from build123d import *

# Parameters (mm, degrees)
SKETCH_1_W               = 15
SKETCH_1_H               = 15
SKETCH_1_W_2             = 13
SKETCH_1_H_2             = 13
EXTRUDE_1_DEPTH          = 570
CUT_EXTRUDE_1_DEPTH      = 10
CUT_EXTRUDE_1_DEPTH_BACK = 571.098675669
SKETCH_2_R               = 1.45
SKETCH_3_R               = 1.5
CUT_EXTRUDE_2_DEPTH      = 571.246657158


with BuildPart() as part:
    # 草图1 → 拉伸-薄壁1 (new body)
    with BuildSketch(Plane(origin=(0, 0, 0), x_dir=(1, 0, 0), z_dir=(0, 1, 0))):
        Rectangle(SKETCH_1_W, SKETCH_1_H)
        Rectangle(SKETCH_1_W_2, SKETCH_1_H_2, mode=Mode.SUBTRACT)
    extrude(amount=EXTRUDE_1_DEPTH)

    # 草图2 → 切除-拉伸1 (cut, two sides: drawn at the far end of the back side and taken through both)
    with BuildSketch(Plane.XY.offset(-CUT_EXTRUDE_1_DEPTH_BACK)):
        with Locations(Location((0, 7.5, 0), (0, 0, 180))):
            Circle(SKETCH_2_R)
        with Locations(Location((0, 22.5, 0), (0, 0, 180))):
            Circle(SKETCH_2_R)
        with Locations(Location((0, 42.5, 0), (0, 0, 180))):
            Circle(SKETCH_2_R)
        with Locations(Location((0, 527.5, 0), (0, 0, 180))):
            Circle(SKETCH_2_R)
        with Locations(Location((0, 547.5, 0), (0, 0, 180))):
            Circle(SKETCH_2_R)
        with Locations(Location((0, 562.5, 0), (0, 0, 180))):
            Circle(SKETCH_2_R)
        with Locations(Location((0, 285, 0), (0, 0, 180))):
            Circle(SKETCH_2_R)
        with Locations(Location((0, 305, 0), (0, 0, 180))):
            Circle(SKETCH_2_R)
        with Locations(Location((0, 265, 0), (0, 0, 180))):
            Circle(SKETCH_2_R)
        with Locations(Location((0, 190, 0), (0, 0, 180))):
            Circle(SKETCH_2_R)
        with Locations(Location((0, 170, 0), (0, 0, 180))):
            Circle(SKETCH_2_R)
        with Locations(Location((0, 230, 0), (0, 0, 180))):
            Circle(SKETCH_2_R)
        with Locations(Location((0, 210, 0), (0, 0, 180))):
            Circle(SKETCH_2_R)
        with Locations(Location((0, 405, 0), (0, 0, 180))):
            Circle(SKETCH_2_R)
        with Locations(Location((0, 385, 0), (0, 0, 180))):
            Circle(SKETCH_2_R)
        with Locations(Location((0, 185, 0), (0, 0, 180))):
            Circle(SKETCH_2_R)
        with Locations(Location((0, 165, 0), (0, 0, 180))):
            Circle(SKETCH_2_R)
        with Locations(Location((0, 325, 0), (0, 0, 180))):
            Circle(SKETCH_2_R)
        with Locations(Location((0, 345, 0), (0, 0, 180))):
            Circle(SKETCH_2_R)
        with Locations(Location((0, 365, 0), (0, 0, 180))):
            Circle(SKETCH_2_R)
    extrude(amount=CUT_EXTRUDE_1_DEPTH + CUT_EXTRUDE_1_DEPTH_BACK, mode=Mode.SUBTRACT)

    # 草图3 → 切除-拉伸2 (cut, through all)
    with BuildSketch(Plane(origin=(7.5, 0, 0), x_dir=(0, 0, -1), z_dir=(1, 0, 0))):
        with Locations((0, 60)):
            Circle(SKETCH_3_R)
        with Locations((0, 100)):
            Circle(SKETCH_3_R)
        with Locations((0, 470)):
            Circle(SKETCH_3_R)
        with Locations((0, 510)):
            Circle(SKETCH_3_R)
        with Locations((0, 140)):
            Circle(SKETCH_3_R)
        with Locations((0, 430)):
            Circle(SKETCH_3_R)
    extrude(amount=-CUT_EXTRUDE_2_DEPTH, mode=Mode.SUBTRACT)


solid = part.part
CAD build for the part. Positions are in the model's coordinates, mm. A direction names the side the tool comes from. Round coordinates to 2 decimals unless told otherwise and drop trailing zeros. Loops run counter-clockwise (first coordinate to the right, second up) from the corner with the lowest first, then second, coordinate; pieces in that order, holes last. Notation, with made-up numbers: M 73.25,-26 L 86.25,-26 A30 cw 86.25,1 Z; hole C 76,32 d4. An arc over 180 degrees is marked long. One line per question, with ' | ' between items. Start each with the question number.
Item 1: Wall check: line 1 (X direction, y = 390, z = -5.5); line 2 (X direction, y = 210, z = 6.8). Give the ranges that are in metal, low to high.
Item 2: Cut at A-A, the plane y = 476.5. Write the cut outline in (x, z), plus the area to 3 significant figures.
Item 3: Which spindle directions (+Z, -Z, +X, -X, +Y, -Y) get a long thin tool onto all of the face, cutting with end or side? Do faces 1 (the flat face through (0, 281, -7.5)), 2 (the flat face through (6.5, 281, 0)). Say none if no direction does.
Item 4: Two-plate mould, pull along X, no slides. Class faces 3 (the flat face through (0, 281, 6.5)), 4 (the flat face through (0, 281, 7.5)), 5 (the flat face through (7.5, 281, 0)): pulls with the +X half, pulls with the -X half, needs draft (parallel to the pull), parting line crosses it, or undercut.
Responses:
1) line 1: x = -7.5 to -6.5, 6.5 to 7.5 | line 2: x = -7.5 to -1.45, 1.45 to 7.5
2) outline: M -7.5,-7.5 L 7.5,-7.5 L 7.5,7.5 L -7.5,7.5 Z; hole M -6.5,-6.5 L 6.5,-6.5 L 6.5,6.5 L -6.5,6.5 Z | area: 56.0 mm²
3) face 1: -Z, +X, -X, +Y, -Y | face 2: +Y, -Y
4) face 3: undercut | face 4: needs draft | face 5: pulls with the +X half
